CAD build for the part. Positions are in the model's coordinates, mm. A direction names the side the tool comes from. Round coordinates to 2 decimals unless told otherwise and drop trailing zeros. Order: outer loops, then holes, each group sorted by start corner. A loop starts at its lowest first (then second) coordinate and runs counter-clockwise, first axis right, second up.
```python
from build123d import *

# Parameters (mm, degrees)
BOSS_EXTRUDE1_DEPTH      = 57.15
BOSS_EXTRUDE1_DEPTH_BACK = 57.15
SKETCH1_W                = 6.35
SKETCH1_H                = 38.1
SKETCH2_R                = 2.1
CUT_EXTRUDE2_DEPTH       = 69.759094853


# Read off the part's stored shape, not the designer's step: Trou taraudé M4x0.71
with BuildPart() as part:
    # Sketch1 → Boss-Extrude1 (new, two sides: drawn at the far end of the back side and taken through both)
    with BuildSketch(Plane.XY.offset(-BOSS_EXTRUDE1_DEPTH_BACK)):
        Rectangle(SKETCH1_W, SKETCH1_H)
    extrude(amount=BOSS_EXTRUDE1_DEPTH + BOSS_EXTRUDE1_DEPTH_BACK)

    # Sketch2 → Cut-Extrude2 (cut, through all)
    with BuildSketch(Plane(origin=(0, 19.05, 0), x_dir=(1, 0, 0), z_dir=(0, 1, 0))):
        with Locations(Location((0, 40.513, 0), (0, 0, 270))):
            Circle(SKETCH2_R)
        with Locations(Location((0, -40.513, 0), (0, 0, 270))):
            Circle(SKETCH2_R)
    extrude(amount=-CUT_EXTRUDE2_DEPTH, mode=Mode.SUBTRACT)

    # Trou taraudé M4x0.71 outline → Trou taraudé M4x0.71 (revolve, cut)
    with BuildSketch(Plane.XZ.offset(12.7)):
        Polygon((0, 41.811742237), (1.65, 41.811742237), (1.65, 56.775), (2.025, 57.15), (0, 57.15), align=None)
    trou_taraud_m4x0_71 = revolve(axis=Axis((0, -12.7, 0), (0, 0, 1)), mode=Mode.SUBTRACT)

    # Trou taraud_ M4x0.71 2 outline → Trou taraud_ M4x0.71 2 (revolve, cut)
    with BuildSketch(Plane.XZ.offset(-12.7)):
        Polygon((0, 41.811742237), (1.65, 41.811742237), (1.65, 56.775), (2.025, 57.15), (0, 57.15), align=None)
    trou_taraud_m4x0_71_2 = revolve(axis=Axis((0, 12.7, 0), (0, 0, 1)), mode=Mode.SUBTRACT)

    # Symétrie1: Trou taraudé M4x0.71, Trou taraud_ M4x0.71 2 across plane
    add(trou_taraud_m4x0_71.mirror(Plane.XY), mode=Mode.SUBTRACT)
    add(trou_taraud_m4x0_71_2.mirror(Plane.XY), mode=Mode.SUBTRACT)


solid = part.part
```
1. Pin check, flat tips, straight feed: P1, Ø2.5, axis at x = 0, y = 12.7, coming from the +Z side; P2, Ø2, axis at x = 0, y = -12.7, coming from the +Z side; P3, Ø2, axis at x = 0, y = -12.7, coming from the -Z side. Stop position of each tip, or through.
2. Mould opens along Z. For faces 4 (the face through (-3.175, 0, -1)), 5 (the face through (0.092, 0.267, 38.415)), 6 (the face through (0, 0, -57.15)) say: released by +Z, released by -Z, zero draft, split by the parting line, or undercut.
3. Cut at A-A, the plane y = 9. Write the cut outline in (x, z) (3 decimals), and give its area (3 significant figures).
4. Tool access for faces 1 (the face through (3.175, 0, -1)), 2 (the face through (-0.215, -11.064, 49.398)), 3 (the face through (-1.31, 11.7, -49.4)): list every direction of +Z, -Z, +X, -X, +Y, -Y with a clear straight run to the whole face (end or side of a thin tool).
5. Drill centre lines: line 1 (Y direction, x = 0, z = -51.5); line 2 (Z direction, x = 0.25, y = -16); line 3 (X direction, y = 12.7, z = 49.75) (3 decimals). Where is each one in solid material? Low to high.
Outcome:
1. P1: stops at z = 38.83
1. P2: stops at z = 38.67
1. P3: stops at z = -38.67
2. face 4: zero draft
2. face 5: undercut
2. face 6: released by -Z
3. outline: (-3.175, -57.15) - (3.175, -57.15) - (3.175, 57.15) - (-3.175, 57.15) - close; hole circle Ø4.2 at (0, -40.513); hole circle Ø4.2 at (0, 40.513)
3. area: 698 mm2
4. face 1: +Z, -Z, +X, +Y, -Y
4. face 2: +Z
4. face 3: -Z
5. line 1: y = -19.05 to -14.35, -11.05 to 11.05, 14.35 to 19.05
5. line 2: z = -57.15 to -42.6, -38.43 to 38.43, 42.6 to 57.15
5. line 3: x = -3.175 to -1.65, 1.65 to 3.175
